Here's the drawing with two shaded views (mm, measured from the low corner). I have some questions. A direction names the side the tool comes from. Coordinates: 2 decimals unless noted, no trailing zeros. Order: outer loops, then holes, each group sorted by start corner. A loop starts at its lowest first (then second) coordinate and runs counter-clockwise, first axis right, second up. Notation, with made-up numbers: (-25.5, -23) - (-5.5, -23) arc R14 cw to (-5.5, -9) - close; hole circle Ø9 at (-5, 7.5). An arc over 180 degrees is marked (long way). Answer as a JSON object with one key per item and string values. Group by question number.
(1) Imagine slicing it at B-B, the plane y = 11.5. Write out the boundary of the cut face in (x, z), and give its area (3 significant figures).
(2) Imagine slicing it at C-C, the plane x = 152.65. Write out the boundary of the cut face in (y, z).
(3) Imagine slicing it at D-D, the plane x = 90. Write out the boundary of the cut face in (y, z).
(4) Imagine slicing it at A-A, the plane z = 65.4. Write out the boundary of the cut face in (x, y), and give its area (3 significant figures).
(5) Will this pin go through, and if not, where does the flat tip stop? P1, Ø20.5, axis at x = 110, z = 44.5, coming from the +Y side.
(6) Which directions (+Z, -Z, +X, -X, +Y, -Y) give clear straight access to the entire face, cutting with the end or side of a thin tool? Please do the marked faces 4 and 5.
(7) Please list where these lines run through material, in increasing order: probe 1 along X at (y, z) = (3.95, 22.6); probe 2 along Z at (x, y) = (152.65, 1.75); probe 3 along X at (y, z) = (11, 67).
(8) We'd pull the mould along X, two halves only. Please class the marked faces 1, 2 and 3: pulls with the +X half, pulls with the -X half, needs draft (parallel to the pull), parting line crosses it, or undercut.
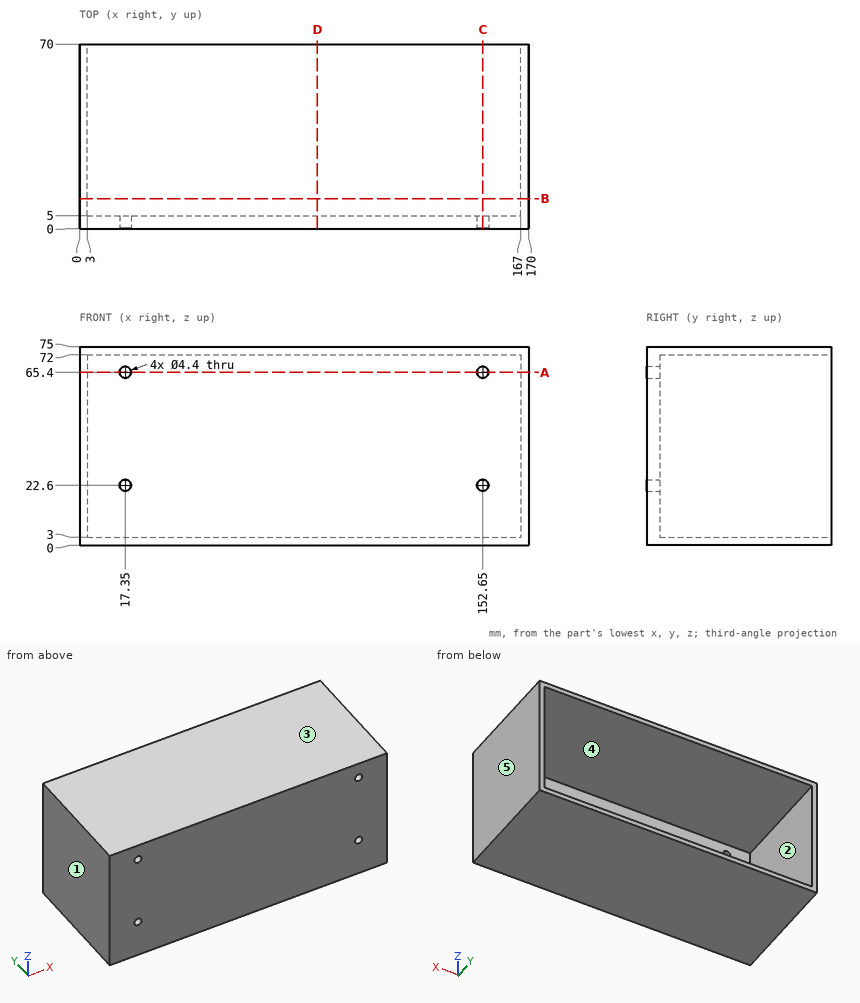
Result set:
{
 "1": {"outline": "(0, 0) - (170, 0) - (170, 75) - (0, 75) - close; hole (3, 3) - (167, 3) - (167, 72) - (3, 72) - close", "area": "1,430 mm^2"},
 "2": {"outline": "(0, 0) - (70, 0) - (70, 3) - (5, 3) - (5, 20.4) - (0, 20.4) - close; (0, 24.8) - (5, 24.8) - (5, 63.2) - (0, 63.2) - close; (0, 67.6) - (5, 67.6) - (5, 72) - (70, 72) - (70, 75) - (0, 75) - close"},
 "3": {"outline": "(0, 0) - (70, 0) - (70, 3) - (5, 3) - (5, 72) - (70, 72) - (70, 75) - (0, 75) - close"},
 "4": {"outline": "(0, 0) - (15.15, 0) - (15.15, 5) - (3, 5) - (3, 70) - (0, 70) - close; (19.55, 0) - (150.45, 0) - (150.45, 5) - (19.55, 5) - close; (154.85, 0) - (170, 0) - (170, 70) - (167, 70) - (167, 5) - (154.85, 5) - close", "area": "1,200 mm^2"},
 "5": {"P1": "stops at y = 5"},
 "6": {"face 4": "+Y", "face 5": "+Z, -Z, +X, +Y, -Y"},
 "7": {"probe 1": "x = 0 to 15.15, 19.55 to 150.45, 154.85 to 170", "probe 2": "z = 0 to 20.4, 24.8 to 63.2, 67.6 to 75", "probe 3": "x = 0 to 3, 167 to 170"},
 "8": {"face 1": "pulls with the -X half", "face 2": "undercut", "face 3": "needs draft"}
}
